Here's the drawing with two shaded views (mm, measured from the low corner). I have some questions. Give positions to 0.01 mm unless a question says otherwise; leave off trailing zeros. Order: outer loops, then holes, each group sorted by start corner. A loop starts at its lowest first (then second) coordinate and runs counter-clockwise, first axis right, second up. Notation, with made-up numbers: M 8,6.5 L 25,6.5 A18 cw 25,15.5 Z; hole C 51.25,-20.75 d9. An arc over 180 degrees is marked long. Use a Markdown table: item, result. Add a question column.
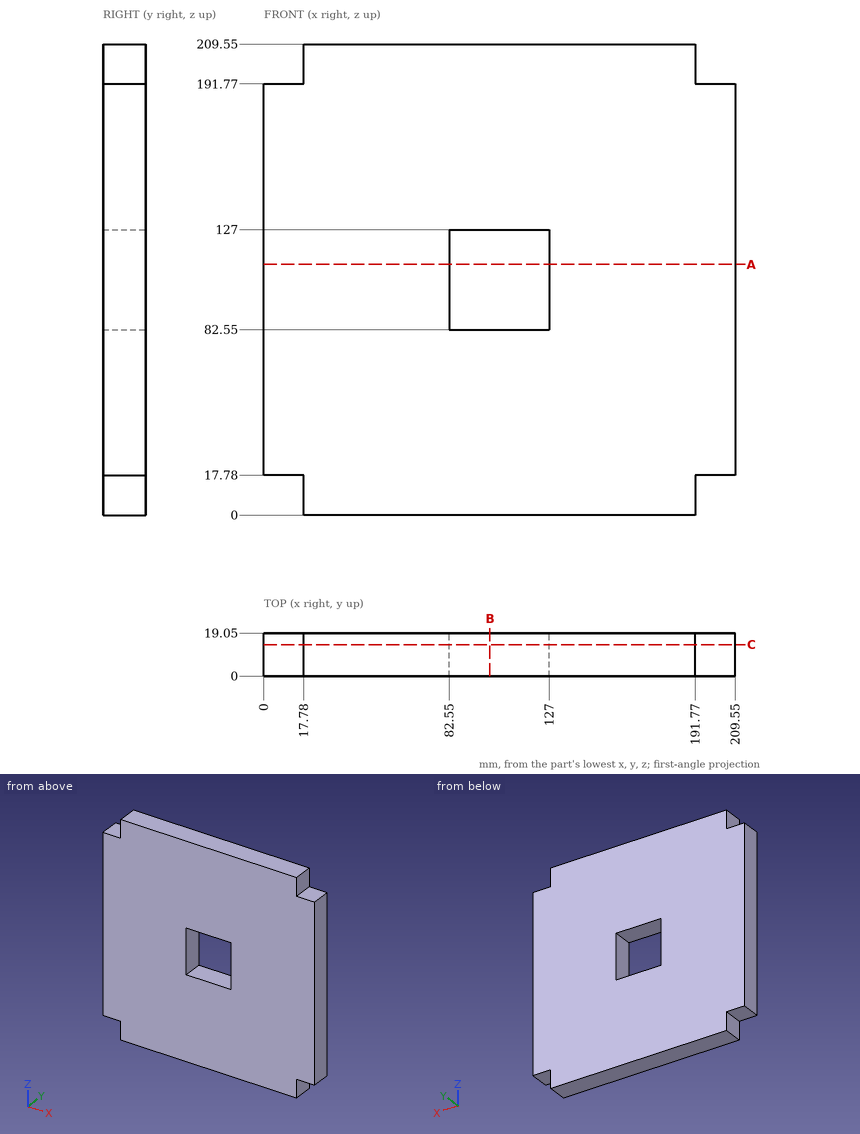
1) Please list where these lines run through material, in increasing order: line 1 (X direction, y = 3.5, z = 115); line 2 (Z direction, x = 195, y = 8.75). Write a range as from..to.
2) For pin 1 (9 mm diameter, centred on y = 10.5, z = 6, fed in from -X); pin 2 (9 mm diameter, centred on x = 6.5, y = 14, fed in from +Z); pin 3 (9 mm diameter, centred on y = 5.5, z = 8, fed in from +X), each with a flat end and sliding along its axis, tell me the tip position at first contact or that it passes through.
3) Suppose I cut it at B-B on x = 100.5. Please give me the cut outline in (y, z).
4) Suppose I cut it at C-C on y = 14. Please give me the cut outline in (x, z).
5) Suppose I cut it at A-A on z = 111.5. Please give me the cut outline in (x, y).
Values found:
| question | item | result |
|---|---|---|
| 1 | line 1 | x = 0..82.55, 127..209.55 |
| 1 | line 2 | z = 17.78..191.77 |
| 2 | pin 1 | stops at x = 17.78 |
| 2 | pin 2 | stops at z = 191.77 |
| 2 | pin 3 | stops at x = 191.77 |
| 3 | outline | M 0,0 L 19.05,0 L 19.05,82.55 L 0,82.55 Z; M 0,127 L 19.05,127 L 19.05,209.55 L 0,209.55 Z |
| 4 | outline | M 0,17.78 L 17.78,17.78 L 17.78,0 L 191.77,0 L 191.77,17.78 L 209.55,17.78 L 209.55,191.77 L 191.77,191.77 L 191.77,209.55 L 17.78,209.55 L 17.78,191.77 L 0,191.77 Z; hole M 82.55,82.55 L 127,82.55 L 127,127 L 82.55,127 Z |
| 5 | outline | M 0,0 L 82.55,0 L 82.55,19.05 L 0,19.05 Z; M 127,0 L 209.55,0 L 209.55,19.05 L 127,19.05 Z |
